from build123d import *

# Parameters (mm, degrees)
SKETCH4_W           = 13.5
SKETCH4_H           = 10.5
BOSS_EXTRUDE2_DEPTH = 2.8
SKETCH5_R           = 3.875
BOSS_EXTRUDE3_DEPTH = 87
SKETCH6_R           = 1.63
CUT_EXTRUDE1_DEPTH  = 90.8
FILLET1_R           = 4


with BuildPart() as part:
    # Sketch4 → Boss-Extrude2 (new body)
    with BuildSketch(Plane.XY):
        with Locations((6.75, 5.25)):
            Rectangle(SKETCH4_W, SKETCH4_H)
    extrude(amount=BOSS_EXTRUDE2_DEPTH)

    # Sketch5 → Boss-Extrude3 (add)
    with BuildSketch(Plane.XY.offset(2.8)):
        with Locations((6.75, 5.25)):
            Circle(SKETCH5_R)
    extrude(amount=BOSS_EXTRUDE3_DEPTH)

    # Sketch6 → Cut-Extrude1 (cut, through all)
    with BuildSketch(Plane.XY.offset(89.8)):
        with Locations((6.75, 5.25)):
            Circle(SKETCH6_R)
    extrude(amount=-CUT_EXTRUDE1_DEPTH, mode=Mode.SUBTRACT)

    # Fillet1
    fillet1_edges = [part.edges().sort_by_distance(p)[0] for p in [
        (0, 10.5, 1.4),
        (13.5, 10.5, 1.4),
        (13.5, 0, 1.4),
        (0, 0, 1.4),
    ]]
    fillet(fillet1_edges, radius=FILLET1_R)


solid = part.part
Here's how the part is built. I have some questions about the finished solid (model axes, mm). A direction names the side the tool comes from. Round coordinates to 2 decimals unless told otherwise and drop trailing zeros. Loops run counter-clockwise (first coordinate to the right, second up) from the corner with the lowest first, then second, coordinate; pieces in that order, holes last. Notation, with made-up numbers: (35, -25) - (90, -25) arc R21 ccw to (90, 5) - close; hole circle Ø6 at (-21, -16). An arc over 180 degrees is marked (long way). One line per question, with ' | ' between items. Start each with the question number.
Q1. I want a section at B-B (y = 5.25). Write out the boundary of the cut face in (x, z) (3 decimals), then the cut area to 3 significant figures.
Q2. We'd pull the mould along Y, two halves only. Please class faces 1 (the cylindrical face through (1.141, 1.203, 1.42)), 2 (the flat face through (13.5, 5, 1)), 3 (the cylindrical face through (8.256, 4.626, 45.529)): +Y half, -Y half, draft (parallel to the pull), parting line (faces both ways), or undercut.
Q3. Please list where these lines run through material, in increasing order: line 1 (Y direction, x = 6.75, z = 22.5) (3 decimals); line 2 (Z direction, x = 11.5, y = 4); line 3 (X direction, y = 5, z = 27.5). Write a range as [from, to].
Q4. I want a section at C-C (z = 16.5). Write out the boundary of the cut face in (x, y) (3 decimals), then the cut area to 3 significant figures.
Q5. For faces 4 (the flat face through (5, 9, 2.8)), 5 (the flat face through (8.2, 4.2, 0)), which set-ups out of +Z, -Z, +X, -X, +Y, -Y let a thin tool reach every point of the face, with its end or its side?
Q6. I want a section at A-A (x = 6.75). Write out the boundary of the cut face in (y, z) (3 decimals), then the cut area to 3 significant figures.
Q7. I want a section at D-D (x = 1). Write out the boundary of the cut face in (y, z), then the cut area to 3 significant figures.
Q8. Will these pins go through, and if not, where does the flat tip stop? pin 1 (2 mm diameter, centred on y = 4.5, z = 47, fed in from -X) (3 decimals); pin 2 (1 mm diameter, centred on x = 7.5, z = 9, fed in from -Y); pin 3 (5 mm diameter, centred on y = 7.5, z = 48, fed in from +X) (3 decimals).
Response values:
1) outline: (0, 0) - (5.12, 0) - (5.12, 89.8) - (2.875, 89.8) - (2.875, 2.8) - (0, 2.8) - close; (8.38, 0) - (13.5, 0) - (13.5, 2.8) - (10.625, 2.8) - (10.625, 89.8) - (8.38, 89.8) - close | area: 419 mm²
2) face 1: -Y half | face 2: draft | face 3: undercut
3) line 1: y = [1.375, 3.62], [6.88, 9.125] | line 2: z = [0, 2.8] | line 3: x = [2.88, 5.14], [8.36, 10.62]
4) outline: circle Ø7.75 at (6.75, 5.25); hole circle Ø3.26 at (6.75, 5.25) | area: 38.8 mm²
5) face 4: +Z | face 5: -Z, +X, -X, +Y, -Y
6) outline: (0, 0) - (3.62, 0) - (3.62, 89.8) - (1.375, 89.8) - (1.375, 2.8) - (0, 2.8) - close; (6.88, 0) - (10.5, 0) - (10.5, 2.8) - (9.125, 2.8) - (9.125, 89.8) - (6.88, 89.8) - close | area: 411 mm²
7) outline: (1.35, 0) - (9.15, 0) - (9.15, 2.8) - (1.35, 2.8) - close | area: 21.8 mm²
8) pin 1: stops at x = 2.875 | pin 2: stops at y = 1.38 | pin 3: stops at x = 10.625
